from build123d import *

# Parameters (mm, degrees)
RESSALTO_EXTRUS_O1_DEPTH = 3
CORTE_EXTRUS_O1_REACH    = 30.32
ESBO_O2_R                = 0.85
RESSALTO_EXTRUS_O2_START = 2.7
ESBO_O4_R                = 3
RESSALTO_EXTRUS_O2_DEPTH = 2.7
CORTE_EXTRUS_O2_REACH    = 30.731
ESBO_O3_R                = 0.5


with BuildPart() as part:
    # Esboço1 → Ressalto-extrusão1 (new body)
    with BuildSketch(Plane.XY):
        with BuildLine():
            Line((-3, 0), (-3, 25))
            ThreePointArc((-3, 25), (0, 28), (3, 25))
            Line((3, 25), (3, 0))
            ThreePointArc((3, 0), (0, -3), (-3, 0))
        make_face()
    extrude(amount=RESSALTO_EXTRUS_O1_DEPTH)

    # Esboço2 → Corte-extrusão1 (cut, up to next)
    with BuildSketch(Plane.XY.offset(3), mode=Mode.PRIVATE) as corte_extrus_o1_sk1:
        Circle(ESBO_O2_R)
    corte_extrus_o1_tool1 = extrude(corte_extrus_o1_sk1.sketch, amount=-CORTE_EXTRUS_O1_REACH, mode=Mode.PRIVATE) & part.part
    add(corte_extrus_o1_tool1.solids().sort_by_distance((0, 0, 3))[0], mode=Mode.SUBTRACT)

    # Esboço4 → Ressalto-extrusão2 (add)
    with BuildSketch(Plane(origin=(0, 0, 0), x_dir=(-1, 0, 0), z_dir=(0, 0, -1)).offset(RESSALTO_EXTRUS_O2_START)):
        with Locations((0, 25)):
            Circle(ESBO_O4_R)
    extrude(amount=-RESSALTO_EXTRUS_O2_DEPTH)

    # Esboço3 → Corte-extrusão2 (cut, up to next)
    with BuildSketch(Plane.XY.offset(3), mode=Mode.PRIVATE) as corte_extrus_o2_sk1:
        with Locations((0, 25)):
            Circle(ESBO_O3_R)
    corte_extrus_o2_tool1 = extrude(corte_extrus_o2_sk1.sketch, amount=-CORTE_EXTRUS_O2_REACH, mode=Mode.PRIVATE) & part.part
    add(corte_extrus_o2_tool1.solids().sort_by_distance((0, 25, 3))[0], mode=Mode.SUBTRACT)


solid = part.part
Here's how the part is built. I have some questions about the finished solid (model axes, mm). A direction names the side the tool comes from. Coordinates: 2 decimals unless noted, no trailing zeros. Loops run counter-clockwise (first coordinate to the right, second up) from the corner with the lowest first, then second, coordinate; pieces in that order, holes last.
1. Imagine slicing it at C-C, the plane z = -0.45. Please give me the cut outline in (x, y), and give its area (3 significant figures).
2. If we mould it in two halves opening along X, with no side actions, what happens to faces 3 (the cylindrical face through (-0.18, -0.83, 1.52)), 4 (the flat face through (-3, 12, 1)), 5 (the cylindrical face through (-0.065, 25.496, 0.19)), 6 (the flat face through (0, 11, 0))? For each: pulls with the +X half, pulls with the -X half, needs draft (parallel to the pull), parting line crosses it, or undercut.
3. Imagine slicing it at D-D, the plane x = -1.8. Please give me the cut outline in (y, z), and give its area (3 significant figures).
4. For faces 1 (the cylindrical face through (0, 28, -1)), 2 (the flat face through (3, 13, 1)), which set-ups out of +Z, -Z, +X, -X, +Y, -Y let a thin tool reach every point of the face, with its end or its side?
5. I need wall thicknesses on L1, parallel to Y at x = 0, z = 1.85; L2, parallel to Z at x = -2.6, y = 19; L3, parallel to Y at x = 0, z = -0.9. Which ranges of each line are inside material? Lowest first, please.
6. For P1, Ø3, axis at x = 0.5, y = 3, coming from the -Z side, with a flat end and sliding along its axis, tell me the tip position at first contact or that it passes through.
7. Imagine slicing it at A-A, the plane x = 0. Please give me the cut outline in (y, z).
8. Imagine slicing it at B-B, the plane z = 0.7. Please give me the cut outline in (x, y), and give its area (3 significant figures).
Taken from the geometry:
1. outline: circle Ø6 at (0, 25); hole circle Ø1 at (0, 25)
1. area: 27.5 mm2
2. face 3: undercut
2. face 4: pulls with the -X half
2. face 5: undercut
2. face 6: needs draft
3. outline: (-2.4, 0) - (22.6, 0) - (22.6, -2.7) - (27.4, -2.7) - (27.4, 3) - (-2.4, 3) - close
3. area: 102 mm2
4. face 1: -Z
4. face 2: +Z, -Z, +X, +Y, -Y
5. L1: y = -3 to -0.85, 0.85 to 24.5, 25.5 to 28
5. L2: z = 0 to 3
5. L3: y = 22 to 24.5, 25.5 to 28
6. P1: stops at z = 0
7. outline: (-3, 0) - (-0.85, 0) - (-0.85, 3) - (-3, 3) - close; (0.85, 0) - (22, 0) - (22, -2.7) - (24.5, -2.7) - (24.5, 3) - (0.85, 3) - close; (25.5, -2.7) - (28, -2.7) - (28, 3) - (25.5, 3) - close
8. outline: (-3, 0) arc R3 ccw to (3, 0) - (3, 25) arc R3 ccw to (-3, 25) - close; hole circle Ø1.7 at (0, 0); hole circle Ø1 at (0, 25)
8. area: 175 mm2
